Autodesk Inventor part; units mm, degrees
ref_plane "YZ Plane" through (0, 0, 0) normal (1, 0, 0) x (0, 1, 0)
ref_plane "XZ Plane" through (0, 0, 0) normal (0, 1, 0) x (-1, 0, 0)
ref_plane "XY Plane" through (0, 0, 0) normal (0, 0, 1) x (1, 0, 0)
sketch "スケッチ1" plane through (0, 0, 0) normal (0, 0, 1) x (1, 0, 0)
  line L0 (0, 16.25) -> (28.465632, 16.25) construction
  line L1 (28.465632, 16.25) -> (28.465632, -16.25) construction
  line L2 (28.465632, -16.25) -> (0, -16.25) construction
  line L3 (0, -16.25) -> (0, 16.25) construction
  line L4 (5, 23.25) -> (-5.158262, 23.25)
  line L5 (-5.158262, 23.25) -> (-34.5, 15.387905)
  line L6 (-34.5, 15.387905) -> (-34.5, -15.387905)
  line L7 (-34.5, -15.387905) -> (-5.158262, -23.25)
  line L8 (-5.158262, -23.25) -> (5, -23.25)
  line L9 (5, -23.25) -> (5, -16.3)
  line L10 (5, -16.3) -> (2.05, -16.3)
  arc A0 (-0.05, -16.3) -> (2.05, -16.3) centre (1, -16.3) ccw
  line L11 (-0.05, -16.3) -> (-0.05, 16.3)
  arc A1 (2.05, 16.3) -> (-0.05, 16.3) centre (1, 16.3) ccw
  line L12 (28.465632, 0) -> (0, 0) construction
  line L13 (2.05, 16.3) -> (5, 16.3)
  line L14 (5, 16.3) -> (5, 23.25)
  line L15 (28.515632, 16.3) -> (-0.05, 16.3) construction
  line L16 (-0.05, 16.3) -> (-0.05, -16.3) construction
  line L17 (-0.05, -16.3) -> (28.515632, -16.3) construction
  line L18 (28.515632, -16.3) -> (28.515632, 16.3) construction
  circle A2 centre (-4.5, 18.25) radius 1.2
  circle A3 centre (-4.5, -18.25) radius 1.2
  line L19 (0, 0) -> (28.465632, 0) construction
  line L20 (2.5, 16.25) -> (2.5, -16.25) construction
  circle A4 centre (-4.5, 18.25) radius 5 construction
  line L21 (-6.087713, 15.5) -> (-7.675426, 18.25)
  line L22 (-7.675426, 18.25) -> (-6.087713, 21)
  line L23 (-6.087713, 21) -> (-2.912287, 21)
  line L24 (-2.912287, 21) -> (-1.324574, 18.25)
  line L25 (-1.324574, 18.25) -> (-2.912287, 15.5)
  line L26 (-2.912287, 15.5) -> (-6.087713, 15.5)
  point P0 (-34.5, 0)
  point P1 (-0.05, 0)
  dimension "d98" = 32.5
  dimension "d100" = 0.05
  dimension "d101" = 1.05
  dimension "d102" = 5
  dimension "d104" = 2.4
  dimension "d106" = 2.5
  dimension "d107" = 7
  dimension "d108" = 18.25
  dimension "d109" = 5
  dimension "d110" = 30
  dimension "d111" = 165
  dimension "d130" = 5.5
extrude "押し出し1" add sketch "スケッチ1" along normal blind 5 contours L14 L13 A1 L11 A0 L10 L9 L8 L7 L6 L5 L4 | L21 L22 L23 L24 L25 L26
sketch "スケッチ6" plane through (0, 0, 0) normal (0, 0, -1) x (-1, 0, 0)
  line L0 (34.5, -15.387905) -> (5.158262, -23.25)
  line L1 (34.5, 15.387905) -> (34.5, -15.387905)
  line L2 (5.158262, 23.25) -> (34.5, 15.387905)
  line L3 (8.5, 17.178203) -> (8.5, -17.178203)
  line L4 (8.5, -17.178203) -> (29.5, -11.55127)
  line L5 (29.5, -11.55127) -> (29.5, 11.55127)
  line L6 (29.5, 11.55127) -> (8.5, 17.178203)
  circle A0 centre (4.5, 18.25) radius 1.2
  point P0 (0, 0)
  dimension "d113" = 5
  dimension "d114" = 5
  dimension "d115" = 5
  dimension "d133" = 4
extrude "押し出し4" cut sketch "スケッチ6" against normal blind 5 contours L6 L5 L4 L3
fillet "フィレット2" radius 1.05 4 edges at (-8.5, 17.1782, 2.5) (-8.5, -17.1782, 2.5) (-29.5, 11.5513, 2.5) (-29.5, -11.5513, 2.5)
sketch "スケッチ7" plane through (0, 0, 0) normal (0, 0, -1) x (-1, 0, 0)
  circle A0 centre (4.5, -18.25) radius 1.2
  circle A1 centre (4.5, 18.25) radius 1.2
  line L0 (2.912287, 15.5) -> (1.324574, 18.25)
  line L1 (1.324574, 18.25) -> (2.912287, 21)
  line L2 (2.912287, 21) -> (6.087713, 21)
  line L3 (6.087713, 21) -> (7.675426, 18.25)
  line L4 (7.675426, 18.25) -> (6.087713, 15.5)
  line L5 (6.087713, 15.5) -> (2.912287, 15.5)
  line L6 (7.6812, 18.25) -> (6.0906, 21.005)
  line L7 (6.0906, 21.005) -> (2.9094, 21.005)
  line L8 (2.9094, 21.005) -> (1.3188, 18.25)
  line L9 (1.3188, 18.25) -> (2.9094, 15.495)
  line L10 (2.9094, 15.495) -> (6.0906, 15.495)
  line L11 (6.0906, 15.495) -> (7.6812, 18.25)
  circle A2 centre (6.6312, 18.25) radius 1.05
  circle A3 centre (5.5656, 20.095673) radius 1.05
  circle A4 centre (3.4344, 20.095673) radius 1.05
  circle A5 centre (2.3688, 18.25) radius 1.05
  circle A6 centre (3.4344, 16.404327) radius 1.05
  circle A7 centre (5.5656, 16.404327) radius 1.05
  line L12 (7.6812, -18.25) -> (6.0906, -21.005)
  line L13 (6.0906, -21.005) -> (2.9094, -21.005)
  line L14 (2.9094, -21.005) -> (1.3188, -18.25)
  line L15 (1.3188, -18.25) -> (2.9094, -15.495)
  line L16 (2.9094, -15.495) -> (6.0906, -15.495)
  line L17 (6.0906, -15.495) -> (7.6812, -18.25)
  circle A8 centre (6.6312, -18.25) radius 1.05
  circle A9 centre (5.5656, -16.404327) radius 1.05
  circle A10 centre (3.4344, -16.404327) radius 1.05
  circle A11 centre (2.3688, -18.25) radius 1.05
  circle A12 centre (3.4344, -20.095673) radius 1.05
  circle A13 centre (5.5656, -20.095673) radius 1.05
  point P0 (0, 0)
  point P1 (6.0906, 21.005)
  point P2 (2.9094, 21.005)
  point P3 (1.3188, 18.25)
  point P4 (2.9094, 15.495)
  point P5 (6.0906, 15.495)
  point P6 (2.9094, -15.495)
  point P7 (2.9094, -21.005)
  point P8 (6.0906, -21.005)
  dimension "d121" = 2.1
  dimension "d119" = 5.5
  dimension "d120" = 0.005
  dimension "d124" = 360
  dimension "d128" = 360
sketch "スケッチ7 outline for 押し出し5" plane through (0, 0, 0) normal (0, 0, -1) x (-1, 0, 0)
  arc A0 (6.6156, 20.095673) -> (5.0406, 21.005) centre (5.5656, 20.095673) ccw
  line L0 (5.0406, 21.005) -> (3.9594, 21.005)
  arc A1 (3.9594, 21.005) -> (2.3844, 20.095673) centre (3.4344, 20.095673) ccw
  line L1 (2.3844, 20.095673) -> (1.8438, 19.159327)
  arc A2 (1.8438, 19.159327) -> (1.8438, 17.340673) centre (2.3688, 18.25) ccw
  line L2 (1.8438, 17.340673) -> (2.3844, 16.404327)
  arc A3 (2.3844, 16.404327) -> (3.9594, 15.495) centre (3.4344, 16.404327) ccw
  line L3 (3.9594, 15.495) -> (5.0406, 15.495)
  arc A4 (5.0406, 15.495) -> (6.6156, 16.404327) centre (5.5656, 16.404327) ccw
  line L4 (6.6156, 16.404327) -> (7.1562, 17.340673)
  arc A5 (7.1562, 17.340673) -> (7.1562, 19.159327) centre (6.6312, 18.25) ccw
  line L5 (7.1562, 19.159327) -> (6.6156, 20.095673)
  arc A6 (6.6156, -16.404327) -> (5.0406, -15.495) centre (5.5656, -16.404327) ccw
  line L6 (3.9594, -15.495) -> (5.0406, -15.495)
  arc A7 (3.9594, -15.495) -> (2.3844, -16.404327) centre (3.4344, -16.404327) ccw
  line L7 (1.8438, -17.340673) -> (2.3844, -16.404327)
  arc A8 (1.8438, -17.340673) -> (1.8438, -19.159327) centre (2.3688, -18.25) ccw
  line L8 (2.3844, -20.095673) -> (1.8438, -19.159327)
  arc A9 (2.3844, -20.095673) -> (3.9594, -21.005) centre (3.4344, -20.095673) ccw
  line L9 (5.0406, -21.005) -> (3.9594, -21.005)
  arc A10 (5.0406, -21.005) -> (6.6156, -20.095673) centre (5.5656, -20.095673) ccw
  line L10 (7.1562, -19.159327) -> (6.6156, -20.095673)
  arc A11 (7.1562, -19.159327) -> (7.1562, -17.340673) centre (6.6312, -18.25) ccw
  line L11 (6.6156, -16.404327) -> (7.1562, -17.340673)
  arc A12 (5.644781, -17.890171) -> (5.384012, -17.438505) centre (4.5, -18.25) ccw
  arc A13 (5.644781, -17.890171) -> (5.644781, -18.609829) centre (6.6312, -18.25) ccw
  arc A14 (5.384012, -19.061495) -> (5.644781, -18.609829) centre (4.5, -18.25) ccw
  arc A15 (5.384012, -19.061495) -> (4.760769, -19.421324) centre (5.5656, -20.095673) ccw
  arc A16 (4.239231, -19.421324) -> (4.760769, -19.421324) centre (4.5, -18.25) ccw
  arc A17 (4.239231, -19.421324) -> (3.615988, -19.061495) centre (3.4344, -20.095673) ccw
  arc A18 (3.355219, -18.609829) -> (3.615988, -19.061495) centre (4.5, -18.25) ccw
  arc A19 (3.355219, -18.609829) -> (3.355219, -17.890171) centre (2.3688, -18.25) ccw
  arc A20 (3.615988, -17.438505) -> (3.355219, -17.890171) centre (4.5, -18.25) ccw
  arc A21 (3.615988, -17.438505) -> (4.239231, -17.078676) centre (3.4344, -16.404327) ccw
  arc A22 (4.760769, -17.078676) -> (4.239231, -17.078676) centre (4.5, -18.25) ccw
  arc A23 (4.760769, -17.078676) -> (5.384012, -17.438505) centre (5.5656, -16.404327) ccw
extrude "押し出し5" cut sketch "スケッチ7 outline for 押し出し5" against normal blind 2
sketch "スケッチ8" plane through (0, 0, 5) normal (0, 0, 1) x (1, 0, 0)
  point P0 (0, 0)
equation "\"d114\" = d113"
equation "\"d115\" = d113"
properties part number "バンパ-" material "アセタール樹脂、黒"
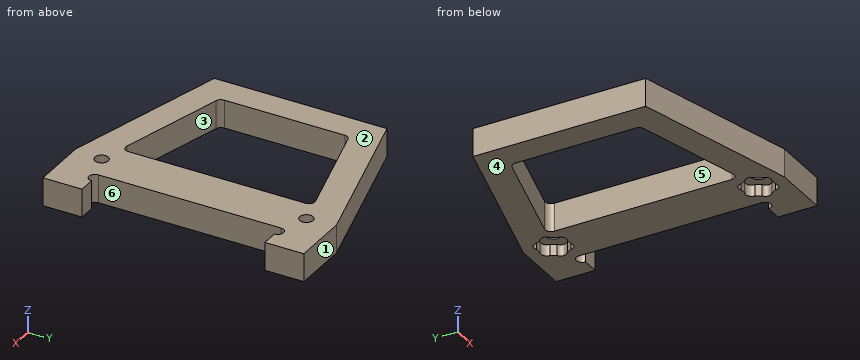
Check sheet for the modelled part. Datum: model origin and axes. Units: mm. Face numbers are marked on the shaded views. A direction names the side the tool comes from. Give positions to 0.01 mm unless a question says otherwise; leave off trailing zeros. Write each loop counter-clockwise with the first axis right and the second up, starting at its lowest first coordinate (ties: lowest second). Pieces come first, ordered by that corner, then holes. Notation, with made-up numbers: (-28, -8) -> (-13, -8) arc R22 ccw to (-13, 4) -> close; hole circle Ø1 at (81, 9). An arc over 180 degrees is marked (long way). Use CSV: the item, a comma, the result in double quotes. Start each with the question number.
Q1. Cross-section at C-C on y = -9. Enter the section's corners in (x, z).
Q2. Scan lines: line 1 along Y through (x, z) = (-4.5, 2.9); line 2 along X through (y, z) = (-7, 3.65); line 3 along Y through (x, z) = (-16, 1.25). Record each from-to range of solid material in increasing order.
Q3. Depth check by flat-ended pin: P1, Ø3, axis at x = -11, y = 3.5, coming from the -Z side; P2, Ø1.5, axis at y = 6.5, z = 3, coming from the +X side; P3, Ø2, axis at x = -16.5, z = 3.5, coming from the +Y side; P4, Ø1.5, axis at x = -27.5, z = 2.5, coming from the -Y side. Enter the tip coordinate at first touch or a pass-through.
Q4. Cross-section at A-A on x = -4.5. Enter the section's corners in (y, z) (3 decimals).
Q5. Cross-section at B-B on z = 3.6. Enter the section's corners in (x, y), and give its area (3 significant figures).
Q6. Cross-section at D-D on x = 1. Enter the section's corners in (y, z), and give its area (3 significant figures).
Q7. Tool access check on the marked faces 4, 5 and 6. Record the directions out of +Z, -Z, +X, -X, +Y, -Y that give a thin tool (end or side, any length) a straight path to the whole face; none if there is none.
Q8. Release check for a two-part mould opening along Y. For the marked faces 1, 2 and 3 record: +Y half, -Y half, draft (parallel to the pull), parting line (faces both ways), or undercut.
Working result:
1,outline,"(-34.5, 0) -> (-29.5, 0) -> (-29.5, 5) -> (-34.5, 5) -> close; (-8.5, 0) -> (-0.05, 0) -> (-0.05, 5) -> (-8.5, 5) -> close"
2,line 1,"y = -23.25 to -19.45, -17.05 to 17.05, 19.45 to 23.25"
2,line 2,"x = -34.5 to -29.5, -8.5 to -0.05"
2,line 3,"y = -20.34 to -15.17, 15.17 to 20.34"
3,P1,"passes through"
3,P2,"stops at x = -0.05"
3,P3,"stops at y = 20.48"
3,P4,"stops at y = -17.46"
4,outline,"(-23.25, 0) -> (-21.005, 0) -> (-21.005, 2) -> (-19.45, 2) -> (-19.45, 5) -> (-23.25, 5) -> close; (-17.05, 2) -> (-15.495, 2) -> (-15.495, 0) -> (15.495, 0) -> (15.495, 2) -> (17.05, 2) -> (17.05, 5) -> (-17.05, 5) -> close; (19.45, 2) -> (21.005, 2) -> (21.005, 0) -> (23.25, 0) -> (23.25, 5) -> (19.45, 5) -> close"
5,outline,"(-34.5, -15.39) -> (-5.16, -23.25) -> (5, -23.25) -> (5, -16.3) -> (2.05, -16.3) arc R1.05 cw to (-0.05, -16.3) -> (-0.05, 16.3) arc R1.05 cw to (2.05, 16.3) -> (5, 16.3) -> (5, 23.25) -> (-5.16, 23.25) -> (-34.5, 15.39) -> close; hole (-29.5, -10.75) arc R1.05 ccw to (-28.72, -11.76) -> (-9.82, -16.82) arc R1.05 ccw to (-8.5, -15.81) -> (-8.5, 15.81) arc R1.05 ccw to (-9.82, 16.82) -> (-28.72, 11.76) arc R1.05 ccw to (-29.5, 10.75) -> close; hole circle Ø2.4 at (-4.5, -18.25); hole circle Ø2.4 at (-4.5, 18.25)"
5,area,"827 mm^2"
6,outline,"(-23.25, 0) -> (-17.35, 0) -> (-17.35, 5) -> (-23.25, 5) -> close; (17.35, 0) -> (23.25, 0) -> (23.25, 5) -> (17.35, 5) -> close"
6,area,"59.0 mm^2"
7,face 4,"-Z, +X, -X, +Y, -Y"
7,face 5,"+Z, -Z"
7,face 6,"+Z, -Z, +X"
8,face 1,"+Y half"
8,face 2,"draft"
8,face 3,"undercut"
